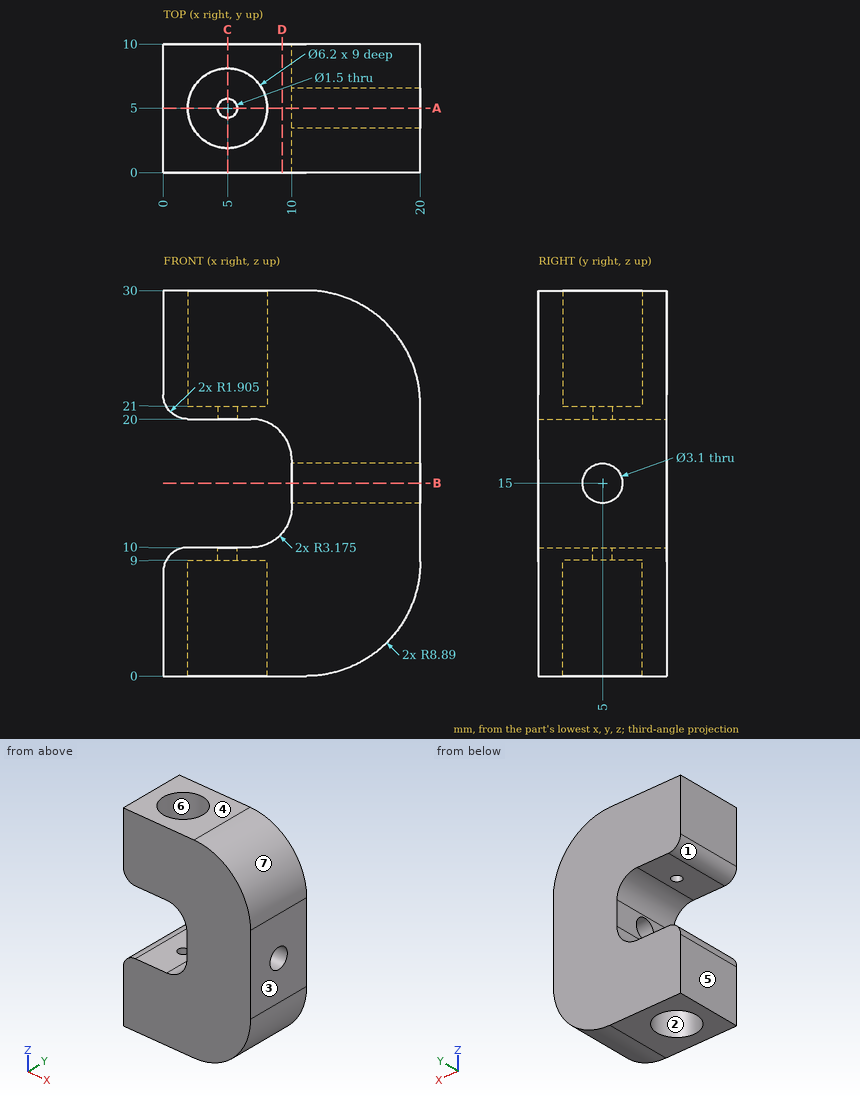
Here's the drawing with two shaded views (mm, measured from the low corner). I have some questions. A direction names the side the tool comes from. Coordinates: 2 decimals unless noted, no trailing zeros. Order: outer loops, then holes, each group sorted by start corner. A loop starts at its lowest first (then second) coordinate and runs counter-clockwise, first axis right, second up.
Item 1: If we section it at A-A, the plane y = 5: Give the number of separate pieces and of enclosed holes in the cut face, then the cut area to 3 significant figures.
Response values:
separate pieces: 4
enclosed holes: 0
area: 323 mm2
Item 2: If we section it at B-B, the plane z = 15: List the corners of the cut face in (x, y) for me, then the cut area to 3 significant figures.
Response values:
outline: (10, 0) - (20, 0) - (20, 3.45) - (10, 3.45) - close; (10, 6.55) - (20, 6.55) - (20, 10) - (10, 10) - close
area: 69.0 mm2
Item 3: If we section it at D-D, the plane x = 9.25: List the corners of the cut face in (y, z) for me.
Response values:
outline: (0, 0) - (10, 0) - (10, 11.13) - (0, 11.13) - close; (0, 18.87) - (10, 18.87) - (10, 30) - (0, 30) - close
Item 4: Thinking about a two-plate mould opening in X: for the marked faces 4, 5, 6 and 7, which applies, pulls with the +X half, pulls with the -X half, needs draft (parallel to the pull), parting line crosses it, or undercut?
Response values:
face 4: needs draft
face 5: pulls with the -X half
face 6: undercut
face 7: pulls with the +X half
Item 5: I'm going to push flat-ended pins straight in: pin 1 Ø2 at (x, y) = (5, 5) entering from -Z; pin 2 Ø1.5 at (y, z) = (6, 24.5) entering from +X; pin 3 Ø3 at (x, y) = (6, 4) entering from +Z. Where does each tip first touch, or does it pass through?
Response values:
pin 1: stops at z = 9
pin 2: stops at x = 19.6
pin 3: stops at z = 21
Item 6: Which directions (+Z, -Z, +X, -X, +Y, -Y) give clear straight access to the entire face, cutting with the end or side of a thin tool? Please do the marked faces 1, 2 and 3.
Response values:
face 1: -X, +Y, -Y
face 2: -Z
face 3: +Z, -Z, +X, +Y, -Y
Item 7: If we section it at C-C, the plane x = 5: List the corners of the cut face in (y, z) for me, then the cut area to 3 significant figures.
Response values:
outline: (0, 0) - (1.9, 0) - (1.9, 9) - (4.25, 9) - (4.25, 10) - (0, 10) - close; (0, 20) - (4.25, 20) - (4.25, 21) - (1.9, 21) - (1.9, 30) - (0, 30) - close; (5.75, 9) - (8.1, 9) - (8.1, 0) - (10, 0) - (10, 10) - (5.75, 10) - close; (5.75, 20) - (10, 20) - (10, 30) - (8.1, 30) - (8.1, 21) - (5.75, 21) - close
area: 85.4 mm2
Item 8: I need wall thicknesses on probe 1 along Z at (x, y) = (2.25, 8.5); probe 2 along Y at (x, z) = (5, 20.7); probe 3 along Y at (x, z) = (14.75, 15). Which ranges of each line are inside material? Lowest first, please.
Response values:
probe 1: z = 0 to 10, 20 to 30
probe 2: y = 0 to 4.25, 5.75 to 10
probe 3: y = 0 to 3.45, 6.55 to 10
